from build123d import *

# Parameters (mm, degrees)
F5_R      = 12
F6_R      = 5
F9_R      = 4.2
F9_R_2    = 3
F10_DEPTH = 28
F11_R     = 3


with BuildPart() as f2:
    # F0 (on Front) → F2 (revolve)
    with BuildSketch(Plane.XZ):
        Polygon((17.75, -7.1372333806), (17.75, -35.1372333806), (19.75, -35.1372333806), (19.75, -5.2919965505), (0, 0), (0, -7.1372333806), align=None)
    revolve(axis=Axis((0, 0, -15.6453922391), (0, 0, -1)))

    # F3 (on Front) → F4 (revolve)
    with BuildSketch(Plane.XZ):
        with BuildLine():
            Line((0, 54.3376104964), (0, -3))
            Line((0, -3), (12, 29.9697290335))
            Line((12, 29.9697290335), (0.906307787, 53.7602287582))
            ThreePointArc((0.906307787, 53.7602287582), (0.5372996083, 54.1810019422), (0, 54.3376104964))
        make_face()
    revolve(axis=Axis((0, 0, 25.6688052482), (0, 0, 1)))

    # F5
    f5_edges = [f2.edges().sort_by_distance(p)[0] for p in [
        (-0.994884, 0, -0.266578),
    ]]
    fillet(f5_edges, radius=F5_R)

    # F6
    f6_edges = [f2.edges().sort_by_distance(p)[0] for p in [
        (-12, 0, 29.969729),
        (-19.75, 0, -5.291997),
    ]]
    fillet(f6_edges, radius=F6_R)

    # F7 (on Front) → F8 (revolve, cut)
    with BuildSketch(Plane.XZ):
        Polygon((3, 45.484368785), (0, 51.9178895465), (0, -35.1372333806), (3, -35.1372333806), (3, 15), (4.8487797808, 15), (10.2698207956, 29.894187778), (5.3315382908, 40.484368785), (3, 40.484368785), align=None)
    revolve(axis=Axis((0, 0, -15.6453922391), (0, 0, -1)), mode=Mode.SUBTRACT)

    # F9 (on face) → F10 (join, through all)
    with BuildSketch(Plane(origin=(0, 0, -35.1372333806), x_dir=(1, 0, 0), z_dir=(0, 0, -1))):
        Circle(F9_R)
        Circle(F9_R_2, mode=Mode.SUBTRACT)
    extrude(amount=-F10_DEPTH)

    # F11
    f11_edges = [f2.edges().sort_by_distance(p)[0] for p in [
        (-17.75, 0, -7.137233),
        (-4.2, 0, -7.137233),
    ]]
    fillet(f11_edges, radius=F11_R)


solid = f2.part
CAD build for the part. Positions are in the model's coordinates, mm. A direction names the side the tool comes from. Round coordinates to 2 decimals unless told otherwise and drop trailing zeros. Order: outer loops, then holes, each group sorted by start corner. A loop starts at its lowest first (then second) coordinate and runs counter-clockwise, first axis right, second up. Notation, with made-up numbers: (15, 85) - (26, 85) arc R28 cw to (26, 121) - close; hole circle Ø6 at (-22, 80). An arc over 180 degrees is marked (long way). Return JSON: item names as keys, results as strings.
(1) Cut at B-B (z = 36). Give the cut face in (x, y).
Answer key:
{"outline": "circle Ø18.38 at (0, 0); hole circle Ø14.85 at (0, 0)"}
(2) Tool access for faces 1 (the face through (-3.848, 17.328, -22.812)), 2 (the face through (18.244, 7.564, -21.951)), 3 (the face through (6.587, -2.731, 16.591)): list every direction of +Z, -Z, +X, -X, +Y, -Y with a clear straight run to the whole face (end or side of a thin tool).
Answer key:
{"face 1": "-Z", "face 2": "+Z, -Z", "face 3": "none"}
(3) Pin check, flat tips, straight feed: pin 1 Ø12 at (x, z) = (-15, 43) entering from +Y; pin 2 Ø3 at (y, z) = (-9.5, 25.5) entering from -X; pin 3 Ø3 at (x, y) = (-8, 13.5) entering from -Z; pin 4 Ø1 at (x, y) = (-9.5, 1) entering from -Z. Stop position of each tip, or through.
Answer key:
{"pin 1": "passes through", "pin 2": "stops at x = -6.8", "pin 3": "stops at z = -8.4", "pin 4": "stops at z = -7.14"}
(4) Wall check: probe 1 along Y at (x, z) = (0, -11.5); probe 2 along Z at (x, y) = (5, 8.5). Give the ranges that are in metal, low to high. Write a range as from..to.
Answer key:
{"probe 1": "y = -19.75..-17.75, -4.2..-3, 3..4.2, 17.75..19.75", "probe 2": "z = -7.14..-1.89, 24.09..28.77, 30.77..34.56"}
(5) Pull direction Z, two halves, no side cores. Call faces 4 (the face through (1.093, -0.344, 49.461)), 5 (the face through (2.824, 5.43, 38.793)), 6 (the face through (4.59, 1.44, 45.39)): +Z half, -Z half, draft (parallel to the pull), parting line (faces both ways), or undercut.
Answer key:
{"face 4": "-Z half", "face 5": "undercut", "face 6": "+Z half"}
(6) Cut at A-A (z = -11). Give the cut face in (x, y).
Answer key:
{"outline": "circle Ø39.5 at (0, 0); circle Ø8.4 at (0, 0); hole circle Ø35.5 at (0, 0); hole circle Ø6 at (0, 0)"}
